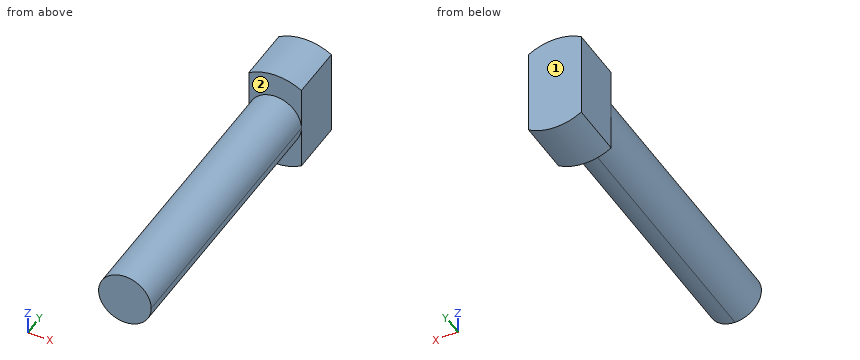
from build123d import *

# Parameters (mm, degrees)
F1_DEPTH = 278.5
F2_DEPTH = 55.5


with BuildPart() as f1:
    # F0 (on Front) → F1 (new body)
    with BuildSketch(Plane.XZ):
        with BuildLine():
            ThreePointArc((-26, -2.27e-08), (-18.3847763028, -18.3847763189), (0, -26))
            ThreePointArc((0, -26), (18.3847763109, -18.3847763109), (26, 0))
            ThreePointArc((26, 0), (18.384776305, 18.3847763167), (-1.64e-08, 26))
            ThreePointArc((-1.64e-08, 26), (-18.3847763247, 18.384776297), (-26, -2.27e-08))
        make_face()
    extrude(amount=F1_DEPTH)

    # F0 (on Front) → F2 (join)
    with BuildSketch(Plane.XZ):
        with BuildLine():
            Line((26, -42.7083130081), (26, -26))
            Line((26, -26), (0, -26))
            Line((0, -26), (-26, -26))
            Line((-26, -26), (-26, -42.7083130081))
            ThreePointArc((-26, -42.7083130081), (0, -50), (26, -42.7083130081))
        make_face()
        with BuildLine():
            Line((0, -26), (26, -26))
            Line((26, -26), (26, 0))
            ThreePointArc((26, 0), (18.3847763109, -18.3847763109), (0, -26))
        make_face()
        with BuildLine():
            Line((-26, -26), (0, -26))
            ThreePointArc((0, -26), (-18.3847763028, -18.3847763189), (-26, -2.27e-08))
            Line((-26, -2.27e-08), (-26, -26))
        make_face()
        with BuildLine():
            ThreePointArc((-26, -2.27e-08), (-18.3847763028, -18.3847763189), (0, -26))
            ThreePointArc((0, -26), (18.3847763109, -18.3847763109), (26, 0))
            ThreePointArc((26, 0), (18.384776305, 18.3847763167), (-1.64e-08, 26))
            ThreePointArc((-1.64e-08, 26), (-18.3847763247, 18.384776297), (-26, -2.27e-08))
        make_face()
        with BuildLine():
            ThreePointArc((-1.64e-08, 26), (18.384776305, 18.3847763167), (26, 0))
            Line((26, 0), (26, 26))
            Line((26, 26), (-1.64e-08, 26))
        make_face()
        with BuildLine():
            Line((-26, 26), (-26, -2.27e-08))
            ThreePointArc((-26, -2.27e-08), (-18.3847763247, 18.384776297), (-1.64e-08, 26))
            Line((-1.64e-08, 26), (-26, 26))
        make_face()
        with BuildLine():
            Line((-1.64e-08, 26), (26, 26))
            Line((26, 26), (26, 42.7083130081))
            ThreePointArc((26, 42.7083130081), (0, 50), (-26, 42.7083130081))
            Line((-26, 42.7083130081), (-26, 26))
            Line((-26, 26), (-1.64e-08, 26))
        make_face()
    extrude(amount=-F2_DEPTH)


solid = f1.part
Check sheet for the modelled part. Datum: model origin and axes. Units: mm. Face numbers are marked on the shaded views. A direction names the side the tool comes from. Give positions to 0.01 mm unless a question says otherwise; leave off trailing zeros. Order: outer loops, then holes, each group sorted by start corner. A loop starts at its lowest first (then second) coordinate and runs counter-clockwise, first axis right, second up. Notation, with made-up numbers: M 6.5,35 L 29.5,35 A29 ccw 29.5,61 Z; hole C 48.5,69 d6. An arc over 180 degrees is marked long. Answer as CSV lines item,"result". Start each with the question number.
Item 1: Cross-section at B-B on x = 16.5. Enter the section's corners in (y, z).
Item 2: Tool access check on the marked faces 1 and 2. Record the directions out of +Z, -Z, +X, -X, +Y, -Y that give a thin tool (end or side, any length) a straight path to the whole face; none if there is none.
Item 3: Cross-section at D-D on y = -77. Enter the section's corners in (x, z).
Item 4: Thickness scan on line 1 (Y direction, x = -21.5, z = -31); line 2 (Z direction, x = -21, y = -260); line 3 (X direction, y = -76, z = -10.5). Record the ranges inside material, lowest first. Write a range as [from, to].
Item 5: Cross-section at C-C on z = 31.5. Enter the section's corners in (x, y).
Item 6: Cross-section at A-A on y = 18.5. Enter the section's corners in (x, z), plus the area to 3 significant figures.
Item 7: Gauge pin test, flat ends, axial feed: P1, Ø5, axis at y = -52, z = -16.5, coming from the -X side; P2, Ø1, axis at x = -13.5, z = 36.5, coming from the -Y side; P3, Ø25, axis at x = -4, z = -26, coming from the -Y side; P4, Ø12, axis at x = 15.5, y = -126.5, coming from the -Z side. Record the tip position at first contact, or that the pin passes through.
Established:
1,outline,"M -278.5,-20.09 L 0,-20.09 L 0,-47.2 L 55.5,-47.2 L 55.5,47.2 L 0,47.2 L 0,20.09 L -278.5,20.09 Z"
2,face 1,"+Z, -Z, +X, -X, +Y"
2,face 2,"+Z, -Y"
3,outline,"C 0,0 d52"
4,line 1,"y = [0, 55.5]"
4,line 2,"z = [-15.33, 15.33]"
4,line 3,"x = [-23.79, 23.79]"
5,outline,"M -26,0 L 26,0 L 26,55.5 L -26,55.5 Z"
6,outline,"M -26,-42.71 A50 ccw 26,-42.71 L 26,42.71 A50 ccw -26,42.71 Z"
6,area,"4,960 mm^2"
7,P1,"stops at x = -21.91"
7,P2,"stops at y = 0"
7,P3,"stops at y = -278.5"
7,P4,"stops at z = -24.2"
